Geometry check sheet. Reference: drawing and pictorial views, mm from the part's lowest x, y, z. A direction names the side the tool comes from. Give positions to 0.01 mm unless a question says otherwise; leave off trailing zeros. Write each loop counter-clockwise with the first axis right and the second up, starting at its lowest first coordinate (ties: lowest second). Pieces come first, ordered by that corner, then holes. Notation, with made-up numbers: M 88,84 L 96,84 A24 ccw 96,99 Z; hole C -1,43.25 d10. An arc over 180 degrees is marked long. One line per item, written item: value. Start each with the question number.
1. Cross-section at C-C on y = 14. Record the cut outline in (x, z).
2. Release check for a two-part mould opening along Y. For the marked faces 3, 4 and 5 record: pulls with the +Y half, pulls with the -Y half, needs draft (parallel to the pull), parting line crosses it, or undercut.
3. Cross-section at B-B on y = 38. Record the cut outline in (x, z), then the cut area to 3 significant figures.
4. Cross-section at A-A on z = 34.5. Record the cut outline in (x, y).
5. Tool access check on the marked faces 1 and 2. Record the directions out of +Z, -Z, +X, -X, +Y, -Y that give a thin tool (end or side, any length) a straight path to the whole face; none if there is none.
6. Gauge pin test, flat ends, axial feed: pin 1 (1.5 mm diameter, centred on x = 25, z = 13.5, fed in from -Y); pin 2 (10 mm diameter, centred on x = 39, z = 10.5, fed in from -Y); pin 3 (1 mm diameter, centred on y = 60, z = 11, fed in from -X) (1 decimal). Record the tip position at first contact, or that the pin passes through.
7. Scan lines: line 1 (Y direction, x = 38, z = 38); line 2 (Z direction, x = 29.5, y = 62); line 3 (Y direction, x = 52, z = 8) (1 decimal). Record each from-to range of solid material in increasing order.
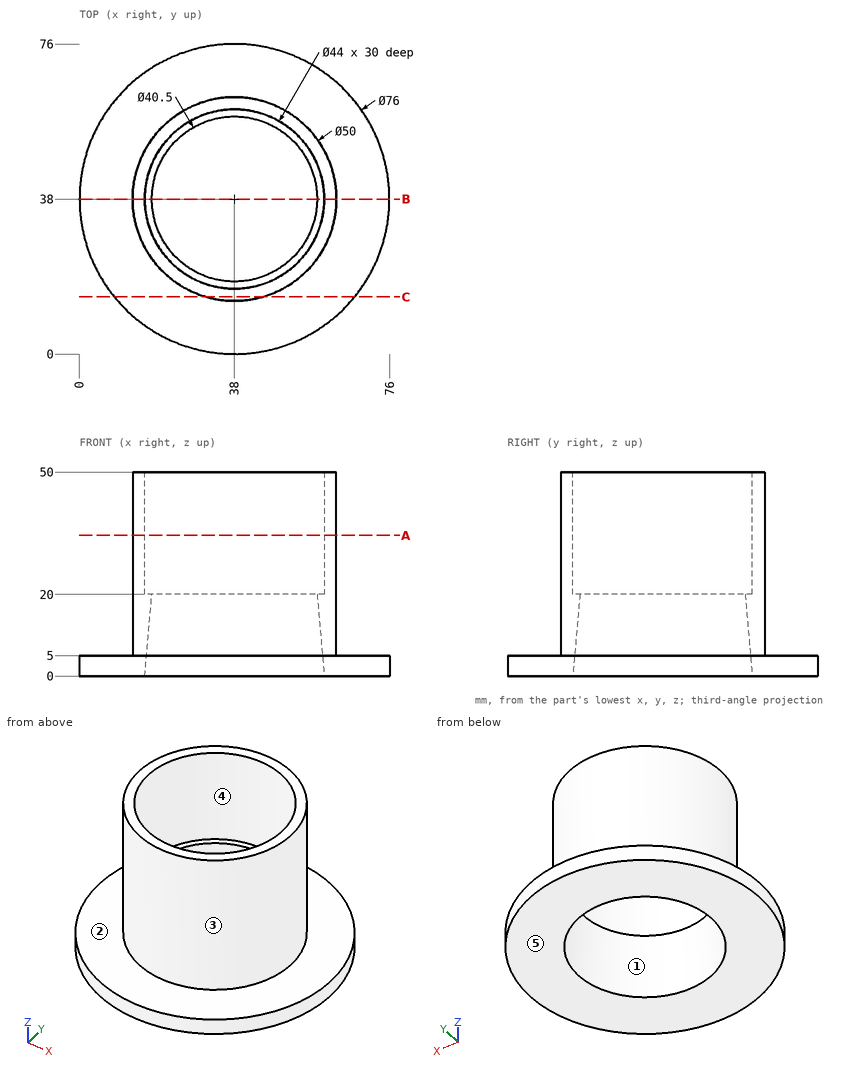
Report:
1. outline: M 8.54,0 L 67.46,0 L 67.46,5 L 45,5 L 45,50 L 31,50 L 31,5 L 8.54,5 Z
2. face 3: parting line crosses it
2. face 4: undercut
2. face 5: needs draft
3. outline: M 0,0 L 16,0 L 17.75,20 L 16,20 L 16,50 L 13,50 L 13,5 L 0,5 Z; M 58.25,20 L 60,0 L 76,0 L 76,5 L 63,5 L 63,50 L 60,50 L 60,20 Z
3. area: 465 mm^2
4. outline: C 38,38 d50; hole C 38,38 d44
5. face 1: -Z
5. face 2: +Z
6. pin 1: stops at y = 16.21
6. pin 2: stops at y = 13
6. pin 3: stops at x = 25.2
7. line 1: y = 13 to 16, 60 to 63
7. line 2: z = 0 to 5
7. line 3: y = 17.3 to 21.9, 54.1 to 58.7
